```python
from build123d import *

# Parameters (mm, degrees)
SKETCH_1_W      = 72.2
SKETCH_1_H      = 14.28
SKETCH_1_R      = 1.5
SKETCH_1_R_2    = 3
EXTRUDE_1_DEPTH = 5
FILLET_1_R      = 2.5
SKETCH_2_R      = 5.5
SKETCH_2_R_2    = 3
EXTRUDE_2_DEPTH = 5
FILLET_2_R      = 1.5


with BuildPart() as part:
    # 草图1 → 凸台-拉伸1 (new body)
    with BuildSketch(Plane.XY):
        Rectangle(SKETCH_1_W, SKETCH_1_H)
        with Locations((31.6, 0)):
            Circle(SKETCH_1_R, mode=Mode.SUBTRACT)
        with Locations((-31.6, 0)):
            Circle(SKETCH_1_R, mode=Mode.SUBTRACT)
        with Locations((10, 0)):
            Circle(SKETCH_1_R_2, mode=Mode.SUBTRACT)
        with Locations((-10, 0)):
            Circle(SKETCH_1_R_2, mode=Mode.SUBTRACT)
    extrude(amount=EXTRUDE_1_DEPTH)

    # 圆角1
    fillet_1_edges = [part.edges().sort_by_distance(p)[0] for p in [
        (-36.1, 7.14, 2.5),
        (36.1, 7.14, 2.5),
        (36.1, -7.14, 2.5),
        (-36.1, -7.14, 2.5),
    ]]
    fillet(fillet_1_edges, radius=FILLET_1_R)

    # 草图2 → 凸台-拉伸2 (add)
    # profile 1 of 2: a face of its own
    with BuildSketch(Plane.XY.offset(5)):
        with Locations((-10, 0)):
            Circle(SKETCH_2_R)
        with Locations((-10, 0)):
            Circle(SKETCH_2_R_2, mode=Mode.SUBTRACT)
    # profile 2 of 2: a face of its own
    with BuildSketch(Plane.XY.offset(5)):
        with Locations((10, 0)):
            Circle(SKETCH_2_R)
        with Locations((10, 0)):
            Circle(SKETCH_2_R_2, mode=Mode.SUBTRACT)
    extrude(amount=EXTRUDE_2_DEPTH)

    # 圆角2
    fillet_2_edges = [part.edges().sort_by_distance(p)[0] for p in [
        (-15.5, 0, 5),
        (4.5, 0, 5),
    ]]
    fillet(fillet_2_edges, radius=FILLET_2_R)


solid = part.part
```
The listing builds one solid part. Answer for the finished solid, in the listing's coordinates (mm). A direction names the side the tool comes from. Give positions to 0.01 mm unless a question says otherwise; leave off trailing zeros. Loops run counter-clockwise (first coordinate to the right, second up) from the corner with the lowest first, then second, coordinate; pieces in that order, holes last. Notation, with made-up numbers: (15.5, 44) - (40.5, 44) arc R27 ccw to (40.5, 79) - close; hole circle Ø3 at (-9.5, -40). An arc over 180 degrees is marked (long way). Return JSON: item names as keys, results as strings. Group by question number.
1. Given pin 1 Ø2 at (x, y) = (-17, 3) entering from +Z; pin 2 Ø1 at (x, z) = (-6.5, 8.5) entering from +Y, each flat-ended and moving along its own axis, determine where each tip first touches the part or whether it passes through.
2. Find section C-C (z = 8.5). Write down the section's boundary in (x, y).
3. Find section D-D (x = 10). Write down the section's boundary in (y, z).
4. Find section A-A (y = 0). State how many separate pieces and enclosed holes the cut face has, then the cut area to 3 significant figures.
5. Determine the mould class of faces 3 (the flat face through (-7.6, -2.4, 10)), 4 (the cylindrical face through (-12.4, -1.8, 4.9)), 5 (the cylindrical face through (35.348, -6.427, 2.535)) for opening direction Y: pulls with the +Y half, pulls with the -Y half, needs draft (parallel to the pull), parting line crosses it, or undercut.
6. Which of the six approach directions +Z, -Z, +X, -X, +Y, -Y give full straight-line access (tool end or side, diameter ignored) to faces 1 (the cylindrical face through (15.08, -2.11, 8.23)), 2 (the flat face through (0, 7.14, 2))?
7. Find section B-B (x = -31.6). Write down the section's boundary in (y, z).
8. Straight lines are drawn through the part: line 1 (Y direction, x = -31.6, z = 3.6); line 2 (Y direction, x = -10, z = 4); line 3 (Z direction, x = -32.5, y = 2.5). For each, find the intervals that lie inside material, in ascending order. Write a range as [from, to].
Verdict:
{
 "1": {"pin 1": "stops at z = 5.05", "pin 2": "stops at y = 4.61"},
 "2": {"outline": "circle Ø11 at (-10, 0); circle Ø11 at (10, 0); hole circle Ø6 at (-10, 0); hole circle Ø6 at (10, 0)"},
 "3": {"outline": "(-7.14, 0) - (-3, 0) - (-3, 10) - (-5.5, 10) - (-5.5, 6.5) arc R1.5 cw to (-7, 5) - (-7.14, 5) - close; (3, 0) - (7.14, 0) - (7.14, 5) - (7, 5) arc R1.5 cw to (5.5, 6.5) - (5.5, 10) - (3, 10) - close"},
 "4": {"separate pieces": "5", "enclosed holes": "0", "area": "323 mm^2"},
 "5": {"face 3": "needs draft", "face 4": "undercut", "face 5": "pulls with the -Y half"},
 "6": {"face 1": "+Z", "face 2": "+Z, -Z, +X, -X, +Y"},
 "7": {"outline": "(-7.14, 0) - (-1.5, 0) - (-1.5, 5) - (-7.14, 5) - close; (1.5, 0) - (7.14, 0) - (7.14, 5) - (1.5, 5) - close"},
 "8": {"line 1": "y = [-7.14, -1.5], [1.5, 7.14]", "line 2": "y = [-7.14, -3], [3, 7.14]", "line 3": "z = [0, 5]"}
}
